from build123d import *

# Parameters (mm, degrees)
TORUS001_R                = 13
CYLINDER001_R             = 4.5
CYLINDER001_DEPTH         = 12
CYLINDER002_R             = 4
CYLINDER002_DEPTH         = 10
PAD001_DEPTH              = 10
BOX_W                     = 8
BOX_H                     = 15.5
BOX_DEPTH                 = 2
CYLINDER004_R             = 2
CYLINDER004_DEPTH         = 7.5
CYLINDER_R                = 2.5
CYLINDER_DEPTH            = 27.5
CYLINDER003_R             = 1.5
CYLINDER003_DEPTH         = 20
CYLINDER016_R             = 4
CYLINDER016_DEPTH         = 2
BOX003_W                  = 4.6
BOX003_H                  = 1.7
BOX003_DEPTH              = 15
FILLET001_R               = 1
BOX002_W                  = 1.7
BOX002_H                  = 4.6
BOX002_DEPTH              = 15
FILLET_R                  = 1
CYLINDER017_R             = 1.5
CYLINDER017_DEPTH         = 10
PAD003_DEPTH              = 2.5
CYLINDER015_R             = 1.5
CYLINDER015_DEPTH         = 11
CYLINDER014_R             = 8
CYLINDER014_DEPTH         = 12
FILLET002_R               = 3
FUSION005_PLACEMENT_ANGLE = 90
CYLINDER012_R             = 16
CYLINDER012_DEPTH         = 20


with BuildPart() as toro001:
    # Torus001 → Torus001 (revolve)
    with BuildSketch(Plane(origin=(55, 0, 11), x_dir=(0, 0, -1), z_dir=(0, -1, 0))):
        with Locations((23, 0)):
            Circle(TORUS001_R)
    revolve(axis=Axis((55, 0, 11), (1, 0, 0)))


with BuildPart() as cilindro001:
    # Cylinder001 → Cylinder001 (new body)
    with BuildSketch(Plane.XY.offset(-6)):
        Circle(CYLINDER001_R)
    extrude(amount=CYLINDER001_DEPTH)


with BuildPart() as cilindro002:
    # Cylinder002 → Cylinder002 (new body)
    with BuildSketch(Plane(origin=(-5, 0, 0), x_dir=(0, 0, -1), z_dir=(1, 0, 0))):
        Circle(CYLINDER002_R)
    extrude(amount=CYLINDER002_DEPTH)


with BuildPart() as pad001:
    # Sketch001 → Pad001 (new body)
    with BuildSketch(Plane.XY):
        with BuildLine():
            ThreePointArc((4.129921, 10.668605), (-0.003253, 15.63264), (-4.128733, 10.662209))
            Line((-5.229172, 10.780737), (-4.128733, 10.662209))
            Line((-5.229172, 16.944185), (-5.229172, 10.780737))
            Line((5.596368, 16.944185), (-5.229172, 16.944185))
            Line((5.596368, 10.638987), (5.596368, 16.944185))
            Line((4.124442, 10.638987), (5.596368, 10.638987))
            Line((4.129921, 10.668605), (4.124442, 10.638987))
        make_face()
    extrude(amount=PAD001_DEPTH)


with BuildPart() as cut:
    # Box → Box (new body)
    with BuildSketch(Plane(origin=(-4, 0, 0), x_dir=(1, 0, 0), z_dir=(0, 0, 1))):
        with Locations((4, 7.75)):
            Rectangle(BOX_W, BOX_H)
    extrude(amount=BOX_DEPTH)

    # Cut: cut Pad001
    add(pad001.part, mode=Mode.SUBTRACT)


with BuildPart() as cilindro004:
    # Cylinder004 → Cylinder004 (new body)
    with BuildSketch(Plane(origin=(0, 12, -6), x_dir=(1, 0, 0), z_dir=(0, 0, 1))):
        Circle(CYLINDER004_R)
    extrude(amount=CYLINDER004_DEPTH)


with BuildPart() as fusion:
    # Cylinder → Cylinder (new body)
    with BuildSketch(Plane.XY.offset(-13.75)):
        Circle(CYLINDER_R)
    extrude(amount=CYLINDER_DEPTH)

    # Fusion: union Cilindro001, Cilindro002, Cut, Cilindro004
    add(cilindro001.part)
    add(cilindro002.part)
    add(cut.part)
    add(cilindro004.part)


with BuildPart() as fusion_1:
    # Fusion placement: moved
    add(fusion.part.moved(Location((27.5, 0, 11))))


with BuildPart() as cylinder003:
    # Cylinder003 → Cylinder003 (new body)
    with BuildSketch(Plane(origin=(23, 0, 11), x_dir=(0, 0, -1), z_dir=(1, 0, 0))):
        Circle(CYLINDER003_R)
    extrude(amount=CYLINDER003_DEPTH)


with BuildPart() as cilindro014:
    # Cylinder016 → Cylinder016 (new body)
    with BuildSketch(Plane.XY.offset(12)):
        Circle(CYLINDER016_R)
    extrude(amount=CYLINDER016_DEPTH)


with BuildPart() as fillet001:
    # Box003 → Box003 (new body)
    with BuildSketch(Plane(origin=(-2.3, -0.85, 22), x_dir=(1, 0, 0), z_dir=(0, 0, 1))):
        with Locations((2.3, 0.85)):
            Rectangle(BOX003_W, BOX003_H)
    extrude(amount=BOX003_DEPTH)

    # Fillet001
    fillet001_edges = [fillet001.edges().sort_by_distance(p)[0] for p in [
        (-2.3, 0, 37),
        (2.3, 0, 37),
    ]]
    fillet(fillet001_edges, radius=FILLET001_R)


with BuildPart() as fusion003:
    # Box002 → Box002 (new body)
    with BuildSketch(Plane(origin=(-0.85, -2.3, 22), x_dir=(1, 0, 0), z_dir=(0, 0, 1))):
        with Locations((0.85, 2.3)):
            Rectangle(BOX002_W, BOX002_H)
    extrude(amount=BOX002_DEPTH)

    # Fillet
    fillet_edges = [fusion003.edges().sort_by_distance(p)[0] for p in [
        (0, -2.3, 37),
        (0, 2.3, 37),
    ]]
    fillet(fillet_edges, radius=FILLET_R)

    # Fusion003: union Fillet001
    add(fillet001.part)


with BuildPart() as fusion003_1:
    # Fusion003 placement: moved
    add(fusion003.part.moved(Location((0, 0, -8))))


with BuildPart() as taladro_tornillo:
    # Cylinder017 → Cylinder017 (new body)
    with BuildSketch(Plane(origin=(0, 0, 4), x_dir=(1, 0, 0), z_dir=(0, 1, 0))):
        Circle(CYLINDER017_R)
    extrude(amount=CYLINDER017_DEPTH)


with BuildPart() as tuerca:
    # Sketch004 → Pad003 (new body)
    with BuildSketch(Plane(origin=(0, 5, -2), x_dir=(1, 0, 0), z_dir=(0, -1, 0))):
        Polygon((0, 9.412578), (-2.887643, 7.71686), (-2.86293, 4.368228), (-2.86293, 0), (2.93707, 0), (2.93707, 4.411033), (2.912357, 7.759665), align=None)
    extrude(amount=PAD003_DEPTH)


with BuildPart() as hueco:
    # Cylinder015 → Cylinder015 (new body)
    with BuildSketch(Plane.XY):
        Circle(CYLINDER015_R)
    extrude(amount=CYLINDER015_DEPTH)

    # Fusion004: union Taladro tornillo, Tuerca
    add(taladro_tornillo.part)
    add(tuerca.part)


with BuildPart() as fusion005:
    # Cylinder014 → Cylinder014 (new body)
    with BuildSketch(Plane.XY):
        Circle(CYLINDER014_R)
    extrude(amount=CYLINDER014_DEPTH)

    # Fillet002
    fillet002_edges = [fusion005.edges().sort_by_distance(p)[0] for p in [
        (-8, 0, 12),
    ]]
    fillet(fillet002_edges, radius=FILLET002_R)

    # Cut003: cut Hueco
    add(hueco.part, mode=Mode.SUBTRACT)

    # Fusion005: union Cilindro014, Fusion003
    add(cilindro014.part)
    add(fusion003_1.part)


with BuildPart() as fusion005_1:
    # Fusion005 placement: moved
    add(fusion005.part.moved(Location((33, 0, 11))).rotate(Axis((33, 0, 11), (0, 1, 0)), FUSION005_PLACEMENT_ANGLE))


with BuildPart() as fusion010:
    # Cylinder012 → Cylinder012 (new body)
    with BuildSketch(Plane(origin=(47, 0, 11), x_dir=(0, 0, -1), z_dir=(1, 0, 0))):
        Circle(CYLINDER012_R)
    extrude(amount=CYLINDER012_DEPTH)

    # Fusion010: union Toro001, Fusion, Cylinder003, Fusion005
    add(toro001.part)
    add(fusion_1.part)
    add(cylinder003.part)
    add(fusion005_1.part)


solid = fusion010.part
Can you work these out from the model? Positions are in its coordinate system, mm. A direction names the side the tool comes from. Give positions to 0.01 mm unless a question says otherwise; leave off trailing zeros. Loops run counter-clockwise (first coordinate to the right, second up) from the corner with the lowest first, then second, coordinate; pieces in that order, holes last. Notation, with made-up numbers: (27, 79.5) - (48, 79.5) arc R35 cw to (48, 116.5) - close; hole circle Ø6 at (50, -26). An arc over 180 degrees is marked (long way). One line per item, written item: value.
(1) If we mould it in two halves opening along Z, with no side actions, what happens to faces 6 (the face through (31.663, -3.549, 9.154)), 7 (the face through (30.4, 14.47, 11.99)), 8 (the face through (35, 2.5, 11))? For each: released by +Z, released by -Z, zero draft, split by the parting line, or undercut.
Verdict:
face 6: split by the parting line
face 7: zero draft
face 8: undercut
(2) If we section it at D-D, the plane x = 59: List the corners of the cut face in (y, z) for me.
Verdict:
outline: circle Ø70.74 at (0, 11)
(3) I need wall thicknesses on line 1 along Z through (x, y) = (37, 1); line 2 along X through (y, z) = (7, 33); line 3 along X through (y, z) = (0.8, 11). Which ranges of each line are inside material? Lowest first, please.
Verdict:
line 1: 3.06 to 9.5, 9.88 to 12.12, 12.5 to 18.94
line 2: 42 to 68
line 3: 22.5 to 43, 44 to 67
(4) If we section it at A-A, the plane x = 27.5: List the corners of the cut face in (y, z) for me, plus the area to 4 significant figures.
Verdict:
outline: (-4.5, 5) - (-2.5, 5) - (-2.5, -2.75) - (2.5, -2.75) - (2.5, 5) - (4.5, 5) - (4.5, 11) - (10, 11) - (10, 5) - (14, 5) - (14, 11) - (15.5, 11) - (15.5, 13) - (4.5, 13) - (4.5, 17) - (2.5, 17) - (2.5, 24.75) - (-2.5, 24.75) - (-2.5, 17) - (-4.5, 17) - close
area: 231.5 mm^2
(5) I'm going to push flat-ended pins straight in: pin 1 (2 mm diameter, centred on y = -2, z = 26, fed in from -X); pin 2 (9 mm diameter, centred on x = 26.5, y = 12, fed in from +Z); pin 3 (4 mm diameter, centred on x = 53.5, y = 28, fed in from -Z); pin 4 (10 mm diameter, centred on y = 18, z = -0.5, fed in from +X). Where does each tip first touch, or does it pass through?
Verdict:
pin 1: x = 43.96
pin 2: z = 13
pin 3: z = -13.8
pin 4: x = 68
(6) If we section it at B-B, the plane x = 37: List the corners of the cut face in (y, z) for me.
Verdict:
outline: (0, 9.5) arc R1.5 ccw to (0, 12.5) - (2.5, 12.5) - (2.5, 13.87) - (5, 13.87) - (5, 12.5) - (7.86, 12.5) arc R8 ccw (long way) to (7.86, 9.5) - (5, 9.5) - (5, 8.07) - (2.5, 8.07) - (2.5, 9.5) - close
(7) If we section it at C-C, the plane x = 48: List the corners of the cut face in (y, z) for me.
Verdict:
outline: circle Ø67.91 at (0, 11)
(8) On a 3-axis mill with a long thin cutter (end or side, diameter ignored), from which of +Z, -Z, +X, -X, +Y, -Y can I reach the whole of each face in a straight line? I mean faces 1 (the face through (27, 0, 24.75)), 2 (the face through (38.464, 6.481, 11.325)), 3 (the face through (34, 4, 13.863)), 4 (the face through (25, 0, 1)), 5 (the face through (67, 0, 11)). Say none if no direction works.
Verdict:
face 1: +Z, -X, +Y, -Y
face 2: +Y
face 3: none
face 4: -Z
face 5: +X
